```python
from build123d import *

# Parameters (mm, degrees)
F0_R     = 1.65
F0_W     = 155.4
F0_H     = 88.4
F1_DEPTH = 3
F2_R     = 2.99999
F3_R     = 1.5


# Not quite as in the source:
# - a fillet or chamfer is up to 0.001 mm smaller than in the source, because OpenCascade refuses the exact size


with BuildPart() as f1:
    # F0 (on Front) → F1 (new body)
    with BuildSketch(Plane.XZ):
        with BuildLine():
            Line((83.5, 64), (-83.5, 64))
            ThreePointArc((-83.5, 64), (-89.5104076401, 61.5104076401), (-92, 55.5))
            Line((-92, 55.5), (-92, -55.5))
            ThreePointArc((-92, -55.5), (-89.5104076401, -61.5104076401), (-83.5, -64))
            Line((-83.5, -64), (83.5, -64))
            ThreePointArc((83.5, -64), (89.5104076401, -61.5104076401), (92, -55.5))
            Line((92, -55.5), (92, 55.5))
            ThreePointArc((92, 55.5), (89.5104076401, 61.5104076401), (83.5, 64))
        make_face()
        with Locations((-78, -58.5)):
            Circle(F0_R, mode=Mode.SUBTRACT)
        with Locations((0, -57)):
            Circle(F0_R, mode=Mode.SUBTRACT)
        with Locations((78, -58.5)):
            Circle(F0_R, mode=Mode.SUBTRACT)
        with BuildLine():
            Line((-83.5, -50.5), (-83.5, 52.5))
            Line((-83.5, 52.5), (83.5, 52.5))
            Line((83.5, 52.5), (83.5, -51.5))
            ThreePointArc((83.5, -51.5), (83.2071067812, -52.2071067812), (82.5, -52.5))
            Line((82.5, -52.5), (47.5, -52.5))
            ThreePointArc((47.5, -52.5), (46.7928932188, -52.2071067812), (46.5, -51.5))
            ThreePointArc((46.5, -51.5), (46.2071067812, -50.7928932188), (45.5, -50.5))
            Line((45.5, -50.5), (-83.5, -50.5))
        make_face(mode=Mode.SUBTRACT)
        with Locations((-78, 56.1)):
            Circle(F0_R, mode=Mode.SUBTRACT)
        with Locations((0, 54.25)):
            Circle(F0_R, mode=Mode.SUBTRACT)
        with Locations((78, 56.1)):
            Circle(F0_R, mode=Mode.SUBTRACT)
        with BuildLine():
            Line((83.5, 52.5), (-83.5, 52.5))
            Line((-83.5, 52.5), (-83.5, -50.5))
            Line((-83.5, -50.5), (45.5, -50.5))
            ThreePointArc((45.5, -50.5), (46.2071067812, -50.7928932188), (46.5, -51.5))
            ThreePointArc((46.5, -51.5), (46.7928932188, -52.2071067812), (47.5, -52.5))
            Line((47.5, -52.5), (82.5, -52.5))
            ThreePointArc((82.5, -52.5), (83.2071067812, -52.2071067812), (83.5, -51.5))
            Line((83.5, -51.5), (83.5, 52.5))
        make_face()
        with Locations((-1.5, 3.7)):
            Rectangle(F0_W, F0_H, mode=Mode.SUBTRACT)
    extrude(amount=F1_DEPTH)

    # F2 (radius 3 in the source; OpenCascade refuses exactly that, so slightly less here)
    f2_edges = [f1.edges().sort_by_distance(p)[0] for p in [
        (92, -3, 0),
    ]]
    fillet(f2_edges, radius=F2_R)

    # F3
    f3_edges = [f1.edges().sort_by_distance(p)[0] for p in [
        (-79.2, -3, 3.7),
        (-1.5, -3, 47.9),
        (76.2, -3, 3.7),
        (-1.5, -3, -40.5),
    ]]
    fillet(f3_edges, radius=F3_R)


solid = f1.part
```
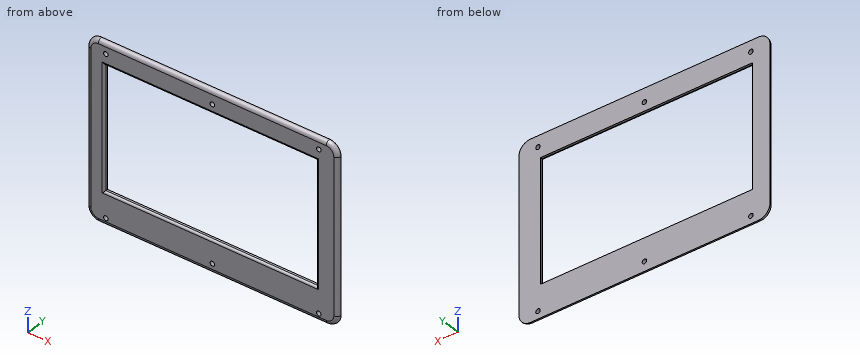
The model under review builds one solid part; all positions refer to its coordinate system, in mm. Give positions to 0.01 mm unless a question says otherwise; leave off trailing zeros. Write each loop counter-clockwise with the first axis right and the second up, starting at its lowest first coordinate (ties: lowest second). Pieces come first, ordered by that corner, then holes. Notation, with made-up numbers: M 49.5,-36 L 59.5,-36 A21 cw 59.5,-30 Z; hole C 51.25,-3.5 d7. An arc over 180 degrees is marked long. Answer in a Markdown table with one row per item.
Item 1: For P1, Ø2.5, axis at x = 0, z = 54.25, coming from the -Y side; P2, Ø1.7, axis at y = -0.5, z = 17, coming from the -X side, all flat-tipped, find the tip position at first contact; note any pin that passes through.
Check sheet entries:
| item | result |
|---|---|
| P1 | through |
| P2 | x = -92 |
Item 2: Add section C-C on y = -1. Give the boundary of the cut face in (x, z), plus the area to 3 significant figures.
Check sheet entries:
| item | result |
|---|---|
| outline | M -91.83,-55.5 A8.33 ccw -83.5,-63.83 L 83.5,-63.83 A8.33 ccw 91.83,-55.5 L 91.83,55.5 A8.33 ccw 83.5,63.83 L -83.5,63.83 A8.33 ccw -91.83,55.5 Z; hole C -78,-58.5 d3.3; hole C -78,56.1 d3.3; hole M -79.2,-40.5 L 76.2,-40.5 L 76.2,47.9 L -79.2,47.9 Z; hole C 0,-57 d3.3; hole C 0,54.25 d3.3; hole C 78,-58.5 d3.3; hole C 78,56.1 d3.3 |
| area | 9,600 mm2 |
Item 3: For line 1 along Z through (x, y) = (-78, -1.7); line 2 along Z through (x, y) = (0, -1.1); line 3 along Z through (x, y) = (-30, -0.25), list the stretches that pass through material, from the lowest coordinate up.
Check sheet entries:
| item | result |
|---|---|
| line 1 | -63.47 to -60.15, -56.85 to -40.51, 47.91 to 54.45, 57.75 to 63.47 |
| line 2 | -63.79 to -58.65, -55.35 to -40.5, 47.9 to 52.6, 55.9 to 63.79 |
| line 3 | -63.99 to -40.5, 47.9 to 63.99 |
